Design review of the part built by this model. Coordinates are the model's own, in mm. Face numbers are marked on the shaded views. Give positions to 0.01 mm unless a question says otherwise; leave off trailing zeros. Order: outer loops, then holes, each group sorted by start corner. A loop starts at its lowest first (then second) coordinate and runs counter-clockwise, first axis right, second up.
```python
from build123d import *

# Parameters (mm, degrees)
F0_W      = 762
F0_H      = 1219.2
F1_DEPTH  = 12.7
F3_W      = 407.9875
F3_H      = 763.5875
F4_DEPTH  = 1.5875
F6_W      = 407.9875
F6_H      = 382.5875
F7_DEPTH  = 1.5875
F9_W      = 280.9875
F9_H      = 573.0875
F10_DEPTH = 1.5875
F12_W     = 280.9875
F12_H     = 573.0875
F13_DEPTH = 1.5875


with BuildPart() as f1:
    # F0 (on Top) → F1 (new body)
    with BuildSketch(Plane.XY):
        Rectangle(F0_W, F0_H)
    extrude(amount=F1_DEPTH)

    # F3 (on face) → F4 (cut)
    with BuildSketch(Plane.XY.offset(12.7)):
        with Locations((151.617306, -202.399241)):
            Rectangle(F3_W, F3_H)
    extrude(amount=-F4_DEPTH, mode=Mode.SUBTRACT)

    # F6 (on face) → F7 (cut)
    with BuildSketch(Plane.XY.offset(12.7)):
        with Locations((151.60625, 392.90625)):
            Rectangle(F6_W, F6_H)
    extrude(amount=-F7_DEPTH, mode=Mode.SUBTRACT)

    # F9 (on face) → F10 (cut)
    with BuildSketch(Plane.XY.offset(12.7)):
        with Locations((-215.10625, -297.65625)):
            Rectangle(F9_W, F9_H)
    extrude(amount=-F10_DEPTH, mode=Mode.SUBTRACT)

    # F12 (on face) → F13 (cut)
    with BuildSketch(Plane.XY.offset(12.7)):
        with Locations((-215.10625, 297.65625)):
            Rectangle(F12_W, F12_H)
    extrude(amount=-F13_DEPTH, mode=Mode.SUBTRACT)


solid = f1.part
```
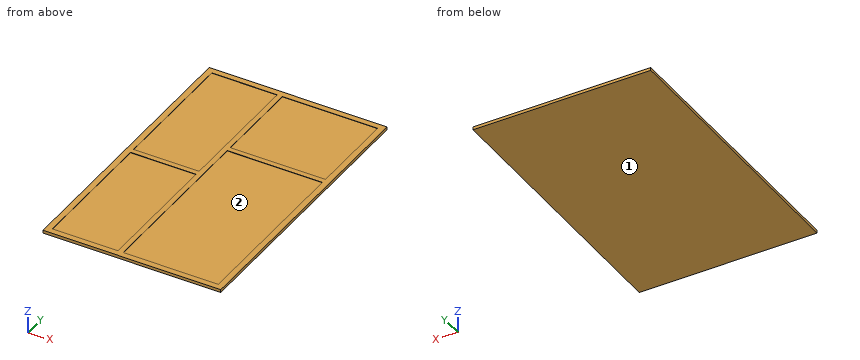
1. For line 1 along Y through (x, z) = (-177, 11.25); line 2 along X through (y, z) = (-391, 12.25); line 3 along Y through (x, z) = (138.5, 11.75), list the stretches that pass through material, from the lowest coordinate up.
Recorded:
line 1: y = -609.6 to -584.2, -11.11 to 11.11, 584.2 to 609.6
line 2: x = -381 to -355.6, -74.61 to -52.38, 355.61 to 381
line 3: y = -609.6 to -584.19, 179.39 to 201.61, 584.2 to 609.6
2. For pin 1 (2 mm diameter, centred on x = -163.5, y = 137, fed in from +Z), flat-tipped, find the tip position at first contact; note if it passes through.
Recorded:
pin 1: stops at z = 11.11
3. Take a section at A-A (y = 293). State the section outline as (x, z) points.
Recorded:
outline: (-381, 0) - (381, 0) - (381, 12.7) - (355.6, 12.7) - (355.6, 11.11) - (-52.39, 11.11) - (-52.39, 12.7) - (-74.61, 12.7) - (-74.61, 11.11) - (-355.6, 11.11) - (-355.6, 12.7) - (-381, 12.7) - close
4. Draft analysis for pull direction Y (two halves, no side actions). For the marked faces 1 and 2, state which applies: pulls with the +Y half, pulls with the -Y half, needs draft (parallel to the pull), parting line crosses it, or undercut.
Recorded:
face 1: needs draft
face 2: undercut
5. Take a section at B-B (x = 71). State the section outline as (y, z) points, then the cut area to 3 significant figures.
Recorded:
outline: (-609.6, 0) - (609.6, 0) - (609.6, 12.7) - (584.2, 12.7) - (584.2, 11.11) - (201.61, 11.11) - (201.61, 12.7) - (179.39, 12.7) - (179.39, 11.11) - (-584.19, 11.11) - (-584.19, 12.7) - (-609.6, 12.7) - close
area: 13,700 mm2
